Autodesk Inventor part; units mm, degrees
ref_plane "YZ Plane" through (0, 0, 0) normal (1, 0, 0) x (0, 1, 0)
ref_plane "XZ Plane" through (0, 0, 0) normal (0, 1, 0) x (-1, 0, 0)
ref_plane "XY Plane" through (0, 0, 0) normal (0, 0, 1) x (1, 0, 0)
ref_plane "Work Plane1" through (39.6605, 279.3484, 58.7085) normal (0, 1, 0) x (1, 0, 0)
sketch "Sketch1" plane through (39.6605, 279.3484, 58.7085) normal (0, 1, 0) x (1, 0, 0)
  line L0 (-19.6605, 58.7085) -> (-19.6605, 78.7085)
  line L1 (-19.6605, 58.7085) -> (-19.6605, 58.7085)
  line L2 (-19.6605, 58.7085) -> (-19.6605, 78.7085)
  line L3 (-19.6605, 78.7085) -> (-19.6605, 78.7085)
  line L4 (-39.6605, 78.7085) -> (-39.6605, 58.7085)
  line L5 (-39.6605, 78.7085) -> (-39.6605, 78.7085)
  line L6 (-39.6605, 78.7085) -> (-39.6605, 58.7085)
  line L7 (-39.6605, 58.7085) -> (-39.6605, 58.7085)
  line L8 (-19.6605, 58.7085) -> (-39.6605, 58.7085)
  line L9 (-39.6605, 58.7085) -> (-39.6605, 53.6285)
  line L10 (-39.6605, 53.6285) -> (-19.6605, 53.6285)
  line L11 (-19.6605, 53.6285) -> (-19.6605, 58.7085)
  dimension "d0" = 5.08
extrude "Extrusion1" add sketch "Sketch1" along normal mid plane 38.1
sketch "Sketch2" plane through (0, 298.3984, 5.08) normal (0, 0, 1) x (1, 0, 0)
  line L0 (20, -38.1) -> (20, 0)
  line L1 (0, 0) -> (20, 0)
  line L2 (0, -38.1) -> (0, 0)
  line L3 (20, -38.1) -> (0, -38.1)
  circle A0 centre (10, -7.62) radius 2.5
  point P0 (0, -298.3984)
  dimension "d3" = 5
  dimension "d6" = 7.62
extrude "Extrusion3" cut sketch "Sketch2" against normal blind 38.1 contours A0
sketch "Sketch3" plane through (0, 260.2984, 5.08) normal (-1, 0, 0) x (0, 0, 1)
  line L0 (-25.08, 298.5016) -> (-5.08, 298.5016)
  line L1 (-25.08, -260.2984) -> (-25.08, 298.5016)
  line L2 (-25.08, -260.2984) -> (-5.08, -260.2984)
  line L3 (-5.08, -260.2984) -> (-5.08, 298.5016)
  line L4 (0, 0) -> (0, 38.1)
  line L5 (-5.08, 38.1) -> (0, 38.1)
  line L6 (-5.08, 0) -> (-5.08, 38.1)
  line L7 (0, 0) -> (-5.08, 0)
  line L8 (0, 38.1) -> (-25.08, 38.1)
  line L9 (-25.08, 38.1) -> (-25.08, 18.1)
  line L10 (-25.08, 18.1) -> (0, 18.1)
  line L11 (0, 18.1) -> (0, 38.1)
  dimension "d11" = 20
extrude "Extrusion4" add sketch "Sketch3" along normal blind 5.08 contours L8 L3 L10 L1 | L5 L4 L10 L3
sketch "Sketch4" plane through (20, 260.2984, 0) normal (1, 0, 0) x (0, 0, -1)
  line L0 (20, 18.1) -> (-5.08, 18.1)
  line L1 (-5.08, 18.1) -> (-5.08, 38.1)
  line L2 (-5.08, 38.1) -> (20, 38.1)
  line L3 (20, 38.1) -> (20, 18.1)
  line L4 (-5.08, 18.1) -> (0, 18.1)
  line L5 (0, 0) -> (0, 18.1)
  line L6 (-5.08, 0) -> (0, 0)
  line L7 (-5.08, 0) -> (-5.08, 18.1)
  point P0 (0, -260.2984)
extrude "Extrusion5" add sketch "Sketch4" along normal blind 5.08
sketch "Sketch5" plane through (0, 260.2984, 0) normal (-1, 0, 0) x (0, 0, 1)
  line L0 (5.08, 18.1) -> (0, 18.1)
  line L1 (0, 0) -> (0, 18.1)
  line L2 (5.08, 0) -> (0, 0)
  line L3 (5.08, 0) -> (5.08, 18.1)
  point P0 (0, -260.2984)
extrude "Extrusion6" add sketch "Sketch5" along normal blind 5.08
sketch "Sketch6" plane through (-5.08, 260.2984, 5.08) normal (-1, 0, 0) x (0, 0, 1)
  line L0 (-25.08, 18.1) -> (-5.08, 18.1)
  line L1 (-5.08, 18.1) -> (-5.08, 0)
  line L2 (-5.08, 0) -> (0, 0)
  line L3 (0, 0) -> (0, 38.1)
  line L4 (0, 38.1) -> (-25.08, 38.1)
  line L5 (-25.08, 38.1) -> (-25.08, 18.1)
  circle A0 centre (-15.08, 28.1) radius 2.5
  point P0 (-5.08, -260.2984)
  dimension "d18" = 5
extrude "Extrusion7" cut sketch "Sketch6" along normal mid plane 2540 contours A0
chamfer "Chamfer1" distance 17.4625 angle 45 2 edges at (-2.54, 278.3984, 0) (22.54, 278.3984, 0)
properties part number "Y belt mount point"
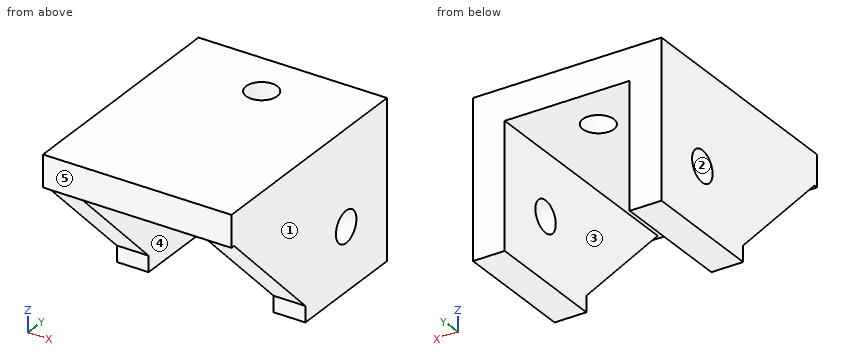
Verification items for the finished model (mm, model axes). Face numbers are marked on the shaded views. A direction names the side the tool comes from. Round coordinates to 2 decimals unless told otherwise and drop trailing zeros. Loops run counter-clockwise (first coordinate to the right, second up) from the corner with the lowest first, then second, coordinate; pieces in that order, holes last. Notation, with made-up numbers: (27, -24.5) -> (72, -24.5) arc R10 ccw to (72, -15.5) -> close; hole circle Ø3 at (-23.5, 58.25). An arc over 180 degrees is marked (long way). Answer as a JSON object with one key per item and string values.
Q1. Scan lines: line 1 (X direction, y = 295.5, z = -6.5); line 2 (Y direction, x = 10, z = 1.7); line 3 (Z direction, x = 17.5, y = 282). Record each from-to range of solid material in increasing order. Write a range as from..to.
Data:
{"line 1": "x = -5.08..0, 20..25.08", "line 2": "y = 260.3..288.28, 293.28..298.4", "line 3": "z = 0..5.08"}
Q2. Go/stop test with flat-tipped pins: P1, Ø8, axis at x = 13.5, z = -2.5, coming from the +Y side; P2, Ø3, axis at y = 288.4, z = -10, coming from the -X side; P3, Ø2, axis at x = -2, z = -18.5, coming from the -Y side; P4, Ø8, axis at x = 10, y = 290.78, coming from the -Z side. Record where each tip stops, or that it passes through.
Data:
{"P1": "stops at y = 298.4", "P2": "passes through", "P3": "stops at y = 278.4", "P4": "stops at z = 0"}
Q3. Access from +Z, -Z, +X, -X, +Y, -Y to the whole of each face (thin tool, end or side, straight path). Record for the marked faces 4 and 5.
Data:
{"face 4": "-Z, +Y, -Y", "face 5": "+Z, -Z, +X, -X, -Y"}
Q4. Section check B-B (z = -16.75). Record the boundary of the cut face in (x, y).
Data:
{"outline": "(-5.08, 277.69) -> (0, 277.69) -> (0, 298.4) -> (-5.08, 298.4) -> close; (20, 277.69) -> (25.08, 277.69) -> (25.08, 298.4) -> (20, 298.4) -> close"}
Q5. Section check D-D (x = 21). Record the boundary of the cut face in (y, z), then the cut area to 3 significant figures.
Data:
{"outline": "(260.3, 0) -> (260.94, 0) -> (278.4, -17.46) -> (278.4, -20) -> (298.4, -20) -> (298.4, 5.08) -> (260.3, 5.08) -> close; hole circle Ø5 at (288.4, -10)", "area": "726 mm2"}
Q6. Section check A-A (x = 10). Record the boundary of the cut face in (y, z).
Data:
{"outline": "(260.3, 0) -> (288.28, 0) -> (288.28, 5.08) -> (260.3, 5.08) -> close; (293.28, 0) -> (298.4, 0) -> (298.4, 5.08) -> (293.28, 5.08) -> close"}
Q7. Draft check along X on the marked faces 1, 2 and 3. Enter one of: pulls with the +X half, pulls with the -X half, needs draft (parallel to the pull), parting line crosses it, or undercut.
Data:
{"face 1": "pulls with the +X half", "face 2": "needs draft", "face 3": "undercut"}
Q8. Section check C-C (y = 279). Record the boundary of the cut face in (x, z), then the cut area to 3 significant figures.
Data:
{"outline": "(-5.08, -20) -> (0, -20) -> (0, 0) -> (20, 0) -> (20, -20) -> (25.08, -20) -> (25.08, 5.08) -> (-5.08, 5.08) -> close", "area": "356 mm2"}
